Source: CAD feature listing. Evaluate the final solid. Frame: model axes, mm. A direction names the side the tool comes from. Coordinates: 2 decimals unless noted, no trailing zeros. Order: outer loops, then holes, each group sorted by start corner. A loop starts at its lowest first (then second) coordinate and runs counter-clockwise, first axis right, second up. Notation, with made-up numbers: (74.5, 79.5) -> (88.5, 79.5) arc R26 ccw to (88.5, 93.5) -> close; hole circle Ø11 at (5.5, 48.25). An arc over 180 degrees is marked (long way). Put each result on its own line as item: value.
from build123d import *

# Parameters (mm, degrees)
SKETCH1_W           = 500
SKETCH1_H           = 450
BOSS_EXTRUDE1_DEPTH = 6
CUT_EXTRUDE1_REACH  = 338.394
SKETCH2_R           = 5
SKETCH3_W           = 20
SKETCH3_H           = 450
BOSS_EXTRUDE2_DEPTH = 30


with BuildPart() as part:
    # Sketch1 → Boss-Extrude1 (new body)
    with BuildSketch(Plane(origin=(0, 0, 0), x_dir=(1, 0, 0), z_dir=(0, 1, 0))):
        Rectangle(SKETCH1_W, SKETCH1_H)
    extrude(amount=BOSS_EXTRUDE1_DEPTH)

    # Sketch2 → Cut-Extrude1 (cut, up to next)
    with BuildSketch(Plane(origin=(0, 6, 0), x_dir=(1, 0, 0), z_dir=(0, 1, 0)), mode=Mode.PRIVATE) as cut_extrude1_sk1:
        with Locations(Location((210, 105, 0), (0, 0, 270))):
            Circle(SKETCH2_R)
    cut_extrude1_tool1 = extrude(cut_extrude1_sk1.sketch, amount=-CUT_EXTRUDE1_REACH, mode=Mode.PRIVATE) & part.part
    # Sketch2 → Cut-Extrude1 (cut, up to next)
    with BuildSketch(Plane(origin=(0, 6, 0), x_dir=(1, 0, 0), z_dir=(0, 1, 0)), mode=Mode.PRIVATE) as cut_extrude1_sk2:
        with Locations(Location((210, -105, 0), (0, 0, 270))):
            Circle(SKETCH2_R)
    cut_extrude1_tool2 = extrude(cut_extrude1_sk2.sketch, amount=-CUT_EXTRUDE1_REACH, mode=Mode.PRIVATE) & part.part
    # Sketch2 → Cut-Extrude1 (cut, up to next)
    with BuildSketch(Plane(origin=(0, 6, 0), x_dir=(1, 0, 0), z_dir=(0, 1, 0)), mode=Mode.PRIVATE) as cut_extrude1_sk3:
        with Locations(Location((210, 0, 0), (0, 0, 270))):
            Circle(SKETCH2_R)
    cut_extrude1_tool3 = extrude(cut_extrude1_sk3.sketch, amount=-CUT_EXTRUDE1_REACH, mode=Mode.PRIVATE) & part.part
    # Sketch2 → Cut-Extrude1 (cut, up to next)
    with BuildSketch(Plane(origin=(0, 6, 0), x_dir=(1, 0, 0), z_dir=(0, 1, 0)), mode=Mode.PRIVATE) as cut_extrude1_sk4:
        with Locations(Location((40, 150, 0), (0, 0, 270))):
            Circle(SKETCH2_R)
    cut_extrude1_tool4 = extrude(cut_extrude1_sk4.sketch, amount=-CUT_EXTRUDE1_REACH, mode=Mode.PRIVATE) & part.part
    # Sketch2 → Cut-Extrude1 (cut, up to next)
    with BuildSketch(Plane(origin=(0, 6, 0), x_dir=(1, 0, 0), z_dir=(0, 1, 0)), mode=Mode.PRIVATE) as cut_extrude1_sk5:
        with Locations(Location((40, 60, 0), (0, 0, 270))):
            Circle(SKETCH2_R)
    cut_extrude1_tool5 = extrude(cut_extrude1_sk5.sketch, amount=-CUT_EXTRUDE1_REACH, mode=Mode.PRIVATE) & part.part
    # Sketch2 → Cut-Extrude1 (cut, up to next)
    with BuildSketch(Plane(origin=(0, 6, 0), x_dir=(1, 0, 0), z_dir=(0, 1, 0)), mode=Mode.PRIVATE) as cut_extrude1_sk6:
        with Locations(Location((40, 0, 0), (0, 0, 270))):
            Circle(SKETCH2_R)
    cut_extrude1_tool6 = extrude(cut_extrude1_sk6.sketch, amount=-CUT_EXTRUDE1_REACH, mode=Mode.PRIVATE) & part.part
    # Sketch2 → Cut-Extrude1 (cut, up to next)
    with BuildSketch(Plane(origin=(0, 6, 0), x_dir=(1, 0, 0), z_dir=(0, 1, 0)), mode=Mode.PRIVATE) as cut_extrude1_sk7:
        with Locations(Location((-110, 150, 0), (0, 0, 270))):
            Circle(SKETCH2_R)
    cut_extrude1_tool7 = extrude(cut_extrude1_sk7.sketch, amount=-CUT_EXTRUDE1_REACH, mode=Mode.PRIVATE) & part.part
    # Sketch2 → Cut-Extrude1 (cut, up to next)
    with BuildSketch(Plane(origin=(0, 6, 0), x_dir=(1, 0, 0), z_dir=(0, 1, 0)), mode=Mode.PRIVATE) as cut_extrude1_sk8:
        with Locations(Location((-110, 30, 0), (0, 0, 270))):
            Circle(SKETCH2_R)
    cut_extrude1_tool8 = extrude(cut_extrude1_sk8.sketch, amount=-CUT_EXTRUDE1_REACH, mode=Mode.PRIVATE) & part.part
    # Sketch2 → Cut-Extrude1 (cut, up to next)
    with BuildSketch(Plane(origin=(0, 6, 0), x_dir=(1, 0, 0), z_dir=(0, 1, 0)), mode=Mode.PRIVATE) as cut_extrude1_sk9:
        with Locations(Location((-110, -30, 0), (0, 0, 270))):
            Circle(SKETCH2_R)
    cut_extrude1_tool9 = extrude(cut_extrude1_sk9.sketch, amount=-CUT_EXTRUDE1_REACH, mode=Mode.PRIVATE) & part.part
    # Sketch2 → Cut-Extrude1 (cut, up to next)
    with BuildSketch(Plane(origin=(0, 6, 0), x_dir=(1, 0, 0), z_dir=(0, 1, 0)), mode=Mode.PRIVATE) as cut_extrude1_sk10:
        with Locations(Location((40, -60, 0), (0, 0, 270))):
            Circle(SKETCH2_R)
    cut_extrude1_tool10 = extrude(cut_extrude1_sk10.sketch, amount=-CUT_EXTRUDE1_REACH, mode=Mode.PRIVATE) & part.part
    # Sketch2 → Cut-Extrude1 (cut, up to next)
    with BuildSketch(Plane(origin=(0, 6, 0), x_dir=(1, 0, 0), z_dir=(0, 1, 0)), mode=Mode.PRIVATE) as cut_extrude1_sk11:
        with Locations(Location((40, -150, 0), (0, 0, 270))):
            Circle(SKETCH2_R)
    cut_extrude1_tool11 = extrude(cut_extrude1_sk11.sketch, amount=-CUT_EXTRUDE1_REACH, mode=Mode.PRIVATE) & part.part
    # Sketch2 → Cut-Extrude1 (cut, up to next)
    with BuildSketch(Plane(origin=(0, 6, 0), x_dir=(1, 0, 0), z_dir=(0, 1, 0)), mode=Mode.PRIVATE) as cut_extrude1_sk12:
        with Locations(Location((-110, -150, 0), (0, 0, 270))):
            Circle(SKETCH2_R)
    cut_extrude1_tool12 = extrude(cut_extrude1_sk12.sketch, amount=-CUT_EXTRUDE1_REACH, mode=Mode.PRIVATE) & part.part
    add(cut_extrude1_tool1.solids().sort_by_distance((210, 6, -105))[0], mode=Mode.SUBTRACT)
    add(cut_extrude1_tool2.solids().sort_by_distance((210, 6, 105))[0], mode=Mode.SUBTRACT)
    add(cut_extrude1_tool3.solids().sort_by_distance((210, 6, 0))[0], mode=Mode.SUBTRACT)
    add(cut_extrude1_tool4.solids().sort_by_distance((40, 6, -150))[0], mode=Mode.SUBTRACT)
    add(cut_extrude1_tool5.solids().sort_by_distance((40, 6, -60))[0], mode=Mode.SUBTRACT)
    add(cut_extrude1_tool6.solids().sort_by_distance((40, 6, 0))[0], mode=Mode.SUBTRACT)
    add(cut_extrude1_tool7.solids().sort_by_distance((-110, 6, -150))[0], mode=Mode.SUBTRACT)
    add(cut_extrude1_tool8.solids().sort_by_distance((-110, 6, -30))[0], mode=Mode.SUBTRACT)
    add(cut_extrude1_tool9.solids().sort_by_distance((-110, 6, 30))[0], mode=Mode.SUBTRACT)
    add(cut_extrude1_tool10.solids().sort_by_distance((40, 6, 60))[0], mode=Mode.SUBTRACT)
    add(cut_extrude1_tool11.solids().sort_by_distance((40, 6, 150))[0], mode=Mode.SUBTRACT)
    add(cut_extrude1_tool12.solids().sort_by_distance((-110, 6, 150))[0], mode=Mode.SUBTRACT)

    # Sketch3 → Boss-Extrude2 (add)
    with BuildSketch(Plane.XZ):
        with Locations((10, 0)):
            Rectangle(SKETCH3_W, SKETCH3_H)
        with Locations((-80, 0)):
            Rectangle(SKETCH3_W, SKETCH3_H)
        with Locations((70, 0)):
            Rectangle(SKETCH3_W, SKETCH3_H)
    extrude(amount=BOSS_EXTRUDE2_DEPTH)


solid = part.part
1. First-contact query: pin 1 (10 mm diameter, centred on y = -21, z = 83.5, fed in from -X); pin 2 (15 mm diameter, centred on y = -20, z = -29.5, fed in from +X); pin 3 (12 mm diameter, centred on x = 38.5, z = 45, fed in from -Y). Flat tips, straight axial feed; report the tip coordinate or a pass-through.
Numbers:
pin 1: stops at x = -90
pin 2: stops at x = 80
pin 3: stops at y = 0
2. Cut plane A-A on y = -11.5. Output: boundary loops of the cut face in (x, z), plus the area to 3 significant figures.
Numbers:
outline: (-90, -225) -> (-70, -225) -> (-70, 225) -> (-90, 225) -> close; (0, -225) -> (20, -225) -> (20, 225) -> (0, 225) -> close; (60, -225) -> (80, -225) -> (80, 225) -> (60, 225) -> close
area: 27,000 mm2
3. Cut plane B-B on z = 86. Output: boundary loops of the cut face in (x, y), plus the area to 3 significant figures.
Numbers:
outline: (-250, 0) -> (-90, 0) -> (-90, -30) -> (-70, -30) -> (-70, 0) -> (0, 0) -> (0, -30) -> (20, -30) -> (20, 0) -> (60, 0) -> (60, -30) -> (80, -30) -> (80, 0) -> (250, 0) -> (250, 6) -> (-250, 6) -> close
area: 4,800 mm2
4. Cut plane C-C on x = -9. Output: boundary loops of the cut face in (y, z).
Numbers:
outline: (0, -225) -> (6, -225) -> (6, 225) -> (0, 225) -> close
5. Set-up query: faces 1 (the flat face through (-35, 0, -3)), 2 (the flat face through (164, 0, -3)), 3 (the flat face through (10, -30, 3)), 4 (the flat face through (-171, 0, -3)). Return all of +Z, -Z, +X, -X, +Y, -Y with unobstructed straight access to the full face (end or side cutting, diameter ignored); none if empty.
Numbers:
face 1: +Z, -Z, -Y
face 2: +Z, -Z, +X, -Y
face 3: +Z, -Z, +X, -X, -Y
face 4: +Z, -Z, -X, -Y
6. Ray query, line 1 along X through (y, z) = (-12, 141.5); line 2 along X through (y, z) = (3.25, 30); line 3 along Y through (x, z) = (-177.5, -94). Return the intervals inside material, ascending.
Numbers:
line 1: x = -90 to -70, 0 to 20, 60 to 80
line 2: x = -250 to -115, -105 to 250
line 3: y = 0 to 6
